from build123d import *

# Parameters (mm, degrees)
SKETCH1_W           = 22
SKETCH1_H           = 22
BOSS_EXTRUDE1_DEPTH = 2
FILLET1_R           = 3
SKETCH2_R           = 1.27
CUT_EXTRUDE1_DEPTH  = 32.176914536
CUT_EXTRUDE2_DEPTH  = 32.176914536
SKETCH4_R           = 5.66890013
CUT_EXTRUDE3_DEPTH  = 10
SKETCH5_W           = 2
SKETCH5_H           = 2
BOSS_EXTRUDE2_DEPTH = 6.68
SKETCH6_W           = 1.502554682
SKETCH6_H           = 1.5
CUT_EXTRUDE4_DEPTH  = 6.8


with BuildPart() as part:
    # Sketch1 → Boss-Extrude1 (new body)
    with BuildSketch(Plane.XY):
        with Locations((11, -11)):
            Rectangle(SKETCH1_W, SKETCH1_H)
    extrude(amount=BOSS_EXTRUDE1_DEPTH)

    # Fillet1
    fillet1_edges = [part.edges().sort_by_distance(p)[0] for p in [
        (0, 0, 1),
        (22, 0, 1),
        (22, -22, 1),
        (0, -22, 1),
    ]]
    fillet(fillet1_edges, radius=FILLET1_R)

    # Sketch2 → Cut-Extrude1 (cut, through all)
    with BuildSketch(Plane.XY.offset(2)):
        with Locations((4.265, -4.265)):
            Circle(SKETCH2_R)
        with Locations((4.265, -17.735)):
            Circle(SKETCH2_R)
        with Locations((17.735, -4.265)):
            Circle(SKETCH2_R)
        with Locations((17.735, -17.735)):
            Circle(SKETCH2_R)
    extrude(amount=-CUT_EXTRUDE1_DEPTH, mode=Mode.SUBTRACT)

    # Sketch3 → Cut-Extrude2 (cut, through all)
    with BuildSketch(Plane.XY.offset(2)):
        with BuildLine():
            Line((7.8, -22), (14.2, -22))
            ThreePointArc((14.2, -22), (11, -18.8), (7.8, -22))
        make_face()
    extrude(amount=-CUT_EXTRUDE2_DEPTH, mode=Mode.SUBTRACT)

    # Sketch4 → Cut-Extrude3 (cut)
    with BuildSketch(Plane.XY.offset(2)):
        with Locations((11, -11)):
            Circle(SKETCH4_R)
    extrude(amount=-CUT_EXTRUDE3_DEPTH, mode=Mode.SUBTRACT)

    # Sketch5 → Boss-Extrude2 (add)
    with BuildSketch(Plane(origin=(0, 0, 0), x_dir=(1, 0, 0), z_dir=(0, 1, 0))):
        with Locations((11, -1)):
            Rectangle(SKETCH5_W, SKETCH5_H)
    extrude(amount=BOSS_EXTRUDE2_DEPTH)

    # Sketch6 → Cut-Extrude4 (cut)
    with BuildSketch(Plane(origin=(0, 6.68, 0), x_dir=(1, 0, 0), z_dir=(0, 1, 0))):
        with Locations((11, -1)):
            Rectangle(SKETCH6_W, SKETCH6_H)
    extrude(amount=-CUT_EXTRUDE4_DEPTH, mode=Mode.SUBTRACT)


solid = part.part
The model under review builds one solid part; all positions refer to its coordinate system, in mm. A direction names the side the tool comes from. Give positions to 0.01 mm unless a question says otherwise; leave off trailing zeros. Loops run counter-clockwise (first coordinate to the right, second up) from the corner with the lowest first, then second, coordinate; pieces in that order, holes last. Notation, with made-up numbers: (-30, 17.5) -> (0, 17.5) arc R22 cw to (0, 29.5) -> close; hole circle Ø4 at (-8.75, 64). An arc over 180 degrees is marked (long way). Answer as a JSON object with one key per item and string values. Group by question number.
Q1. Wall thickness on line 1 along X through (y, z) = (-4.25, 0.3); line 2 along X through (y, z) = (5, 0.8); line 3 along X through (y, z) = (-20.5, 1.45): over which ranges is each line inside the solid? List them lowest first.
Q2. Draft analysis for pull direction Z (two halves, no side actions). For faces 4 (the cylindrical face through (0.86, -21.1, 1.01)), 5 (the flat face through (10.249, 3, 1)), 6 (the flat face through (11, -4, 2)), state which applies: pulls with the +Z half, pulls with the -Z half, needs draft (parallel to the pull), parting line crosses it, or undercut.
Q3. Take a section at D-D (x = 3.75). Write out the cut boundary in (y, z).
Q4. Take a section at A-A (y = 2.5). Write out the cut boundary in (x, z), plus the area to 3 significant figures.
Q5. Take a section at C-C (y = -11). Write out the cut boundary in (x, z).
Q6. Insertion check: pin 1 (0.8 mm diameter, centred on y = 2.5, z = 1.5, fed in from -X); pin 2 (1 mm diameter, centred on x = 9, y = -14, fed in from -Z); pin 3 (1 mm diameter, centred on x = 7, z = 1.5, fed in from +Y); pin 4 (4 mm diameter, centred on x = 4.265, y = -4.265, fed in from -Z). Each pin has a flat end and moves straight along its axis. Give the tip position at first contact, or say it passes through.
Q7. Tool access review of faces 1 (the flat face through (12, 3, 1)), 2 (the flat face through (6, 0, 1)), 3 (the flat face through (0, -11, 1)): name each direction out of +Z, -Z, +X, -X, +Y, -Y from which nothing blocks a thin tool from reaching the whole face with its end or side.
Q8. Take a section at B-B (x = 11). Write out the cut boundary in (y, z).
Answer below:
{
 "1": {"line 1": "x = 0 to 3, 5.53 to 16.47, 19 to 22", "line 2": "x = 10 to 10.25, 11.75 to 12", "line 3": "x = 0.4 to 8.17, 13.83 to 21.6"},
 "2": {"face 4": "needs draft", "face 5": "undercut", "face 6": "pulls with the +Z half"},
 "3": {"outline": "(-22, 0) -> (-18.9, 0) -> (-18.9, 2) -> (-22, 2) -> close; (-16.57, 0) -> (-5.43, 0) -> (-5.43, 2) -> (-16.57, 2) -> close; (-3.1, 0) -> (0, 0) -> (0, 2) -> (-3.1, 2) -> close"},
 "4": {"outline": "(10, 0) -> (12, 0) -> (12, 2) -> (10, 2) -> close; hole (10.25, 0.25) -> (11.75, 0.25) -> (11.75, 1.75) -> (10.25, 1.75) -> close", "area": "1.75 mm2"},
 "5": {"outline": "(0, 0) -> (5.33, 0) -> (5.33, 2) -> (0, 2) -> close; (16.67, 0) -> (22, 0) -> (22, 2) -> (16.67, 2) -> close"},
 "6": {"pin 1": "stops at x = 10", "pin 2": "passes through", "pin 3": "stops at y = 0", "pin 4": "stops at z = 0"},
 "7": {"face 1": "+Z, -Z, +X, +Y", "face 2": "+Z, -Z, -X, +Y", "face 3": "+Z, -Z, -X, +Y, -Y"},
 "8": {"outline": "(-18.8, 0) -> (-16.67, 0) -> (-16.67, 2) -> (-18.8, 2) -> close; (-5.33, 0) -> (6.68, 0) -> (6.68, 0.25) -> (-0.12, 0.25) -> (-0.12, 1.75) -> (6.68, 1.75) -> (6.68, 2) -> (-5.33, 2) -> close"}
}
